Design review of the part built by this model. Coordinates are the model's own, in mm. Coordinates: 2 decimals unless noted, no trailing zeros. Loops run counter-clockwise (first coordinate to the right, second up) from the corner with the lowest first, then second, coordinate; pieces in that order, holes last. Notation, with made-up numbers: (-23, 75) -> (-5, 75) arc R27 ccw to (-5, 114) -> close; hole circle Ø1 at (-39.5, -9). An arc over 180 degrees is marked (long way). Use one line per item in the form item = value. Start each with the question number.
1. For pin 1 (3 mm diameter, centred on x = -90.54, z = 52.27, fed in from -Y); pin 2 (1 mm diameter, centred on y = 3, z = -31.5, fed in from +X), all flat-tipped, find the tip position at first contact; note any pin that passes through.
2. Wall thickness on line 1 (Z direction, x = 117.95, y = 0.9); line 2 (X direction, y = 2.35, z = 13); line 3 (X direction, y = 1.15, z = -58.5): over which ranges is each line inside the solid? List them lowest first. Write a range as from..to.
3. Consider section A-A (z = -68). State the section outline as (x, y) points (3 decimals).
4. Consider section C-C (y = 2.5). State how many separate pieces and enclosed holes the cut face has, then the cut area to 3 significant figures.
5. The part is to be moulded in two halves that separate along Z. For faces 1 (the face through (1.93, 1.565, -107.933)), 2 (the face through (74.96, 1.57, 47.79)), 3 (the face through (-92, 3.175, -9)), say which applies: released by +Z, released by -Z, zero draft, split by the parting line, or undercut.
6. Consider section B-B (x = 5.5). State the section outline as (y, z) points (3 decimals).
from build123d import *

# Parameters (mm, degrees)
SKETCH1_R              = 107.95
SKETCH1_R_2            = 88.9
BOSS_EXTRUDE1_DEPTH    = 3.175
M3_CLEARANCE_HOLE1_D   = 3.2
CIRPATTERN1_COUNT      = 12
BOSS_EXTRUDE2_DEPTH    = 3.175
F_10_CLEARANCE_HOLE3_D = 4.9784
FILLET1_R              = 10
FILLET1_OF_MIRROR1_R   = 10


with BuildPart() as part:
    # Sketch1 → Boss-Extrude1 (new body)
    with BuildSketch(Plane(origin=(0, 0, 0), x_dir=(1, 0, 0), z_dir=(0, 1, 0))):
        with Locations(Location((0, 0, 0), (0, 0, 270))):
            Circle(SKETCH1_R)
        with Locations(Location((0, 0, 0), (0, 0, 270))):
            Circle(SKETCH1_R_2, mode=Mode.SUBTRACT)
    extrude(amount=BOSS_EXTRUDE1_DEPTH)

    # M3 Clearance Hole1 (through all)
    with Locations(Plane(origin=(0, 3.175, 0), x_dir=(1, 0, 0), z_dir=(0, 1, 0))):
        with Locations((0, 104.55)):
            m3_clearance_hole1 = Hole(M3_CLEARANCE_HOLE1_D / 2)

    # CirPattern1: M3 Clearance Hole1 ×12 about axis
    cirpattern1_axis = Axis((0, 0, 0), (0, 1, 0))
    for i in range(1, CIRPATTERN1_COUNT):
        add(m3_clearance_hole1.rotate(cirpattern1_axis, i * 360 / CIRPATTERN1_COUNT), mode=Mode.SUBTRACT)

    # Sketch2 → Boss-Extrude2 (add)
    with BuildSketch(Plane(origin=(0, 0, 0), x_dir=(1, 0, 0), z_dir=(0, 1, 0))):
        with BuildLine():
            Line((-156.234271247, 24.142135624), (-105.215777275, 24.142135624))
            ThreePointArc((-105.215777275, 24.142135624), (-107.95, 0), (-105.215777275, -24.142135624))
            Line((-105.215777275, -24.142135624), (-156.234271247, -24.142135624))
            Line((-156.234271247, -24.142135624), (-156.234271247, 24.142135624))
        make_face()
    boss_extrude2 = extrude(amount=BOSS_EXTRUDE2_DEPTH)

    # #10 Clearance Hole3 (through all)
    with Locations(Plane(origin=(0, 3.175, 0), x_dir=(1, 0, 0), z_dir=(0, 1, 0))):
        with Locations((-132.092135624, -14.142135624), (-117.95, 0), (-132.092135624, 14.142135624), (-146.234271247, 0)):
            f_10_clearance_hole3 = Hole(F_10_CLEARANCE_HOLE3_D / 2)

    # Fillet1
    fillet1_edges = [part.edges().sort_by_distance(p)[0] for p in [
        (-156.234271247, 1.5875, -24.142135624),
        (-156.234271247, 1.5875, 24.142135624),
        (-105.215777275, 1.5875, 24.142135624),
        (-105.215777275, 1.5875, -24.142135624),
    ]]
    fillet(fillet1_edges, radius=FILLET1_R)

    # Mirror1: Boss-Extrude2, #10 Clearance Hole3 across plane
    add(boss_extrude2.mirror(Plane(origin=(0, 0, 0), x_dir=(0, 0, 1), z_dir=(1, 0, 0))))
    add(f_10_clearance_hole3.mirror(Plane(origin=(0, 0, 0), x_dir=(0, 0, 1), z_dir=(1, 0, 0))), mode=Mode.SUBTRACT)

    # Fillet1 of Mirror1
    fillet1_of_mirror1_edges = [part.edges().sort_by_distance(p)[0] for p in [
        (156.234271247, 1.5875, -24.142135624),
        (156.234271247, 1.5875, 24.142135624),
        (105.215777275, 1.5875, 24.142135624),
        (105.215777275, 1.5875, -24.142135624),
    ]]
    fillet(fillet1_of_mirror1_edges, radius=FILLET1_OF_MIRROR1_R)


solid = part.part
Geometry check:
q1.pin_1 = through
q1.pin_2 = 103.41
q2.line_1 = -24.14..-2.49, 2.49..24.14
q2.line_2 = -156.23..-134.3, -129.88..-87.94, 87.94..129.88, 134.3..156.23
q2.line_3 = -90.72..-66.94, 66.94..90.72
q3.outline = (-83.84, 0) -> (-57.264, 0) -> (-57.264, 3.175) -> (-83.84, 3.175) -> close; (57.264, 0) -> (83.84, 0) -> (83.84, 3.175) -> (57.264, 3.175) -> close
q4.separate_pieces = 1
q4.enclosed_holes = 21
q4.area = 16,200 mm²
q5.face_1 = released by -Z
q5.face_2 = undercut
q5.face_3 = zero draft
q6.outline = (0, -107.81) -> (3.175, -107.81) -> (3.175, -88.73) -> (0, -88.73) -> close; (0, 88.73) -> (3.175, 88.73) -> (3.175, 107.81) -> (0, 107.81) -> close
